Part model, mm, in its own coordinate system. Face numbers are marked on the shaded views. A direction names the side the tool comes from. Give positions to 0.01 mm unless a question says otherwise; leave off trailing zeros. Order: outer loops, then holes, each group sorted by start corner. A loop starts at its lowest first (then second) coordinate and runs counter-clockwise, first axis right, second up.
1. Slice it at C-C on z = 6.75. List the corners of the cut face in (x, y), and give its area (3 significant figures).
2. Slice it at A-A on y = 0. List the corners of the cut face in (x, z).
3. Slice it at B-B on x = 38. List the corners of the cut face in (y, z), and give its area (3 significant figures).
4. Probe line 1 (Y direction, x = 43.5, z = 24.5); line 2 (Z direction, x = 40.5, y = 1.55); line 3 (Z direction, x = 48, y = -2.25). List the from-to ranges inside material, lowest first.
5. Which spindle directions (+Z, -Z, +X, -X, +Y, -Y) get a long thin tool onto all of the face, cutting with end or side? Do the marked faces 1 and 2. Say none if no direction does.
6. Drop flat-ended pins along their axis: pin 1 Ø3 at (y, z) = (1.5, 11) entering from -X; pin 2 Ø3 at (y, z) = (-1.5, 17) entering from +X; pin 3 Ø3 at (x, y) = (14.5, 1.5) entering from +Z. Give the stop position or say it passes through.
from build123d import *

# Parameters (mm, degrees)
F1_R     = 2.5
F3_SIZE2 = 0.5
F3_SIZE  = 0.5


with BuildPart() as f2:
    # F2: sweep along a path in F0
    with BuildLine(Plane.XZ) as f2_path:
        Line((0, 0), (0, 10))
        ThreePointArc((0, 10), (4.686291501, 21.313708499), (16, 26))
        Line((16, 26), (96, 26))
    # F1 (on Top) → F2 (sweep)
    with BuildSketch(Plane.XY):
        Circle(F1_R)
    sweep(path=f2_path.line)

    # F3
    f3_edges = [f2.edges().sort_by_distance(p)[0] for p in [
        (-2.5, 0, 0),
        (96, 0, 28.5),
    ]]
    chamfer(f3_edges, length=F3_SIZE, length2=F3_SIZE2)


solid = f2.part
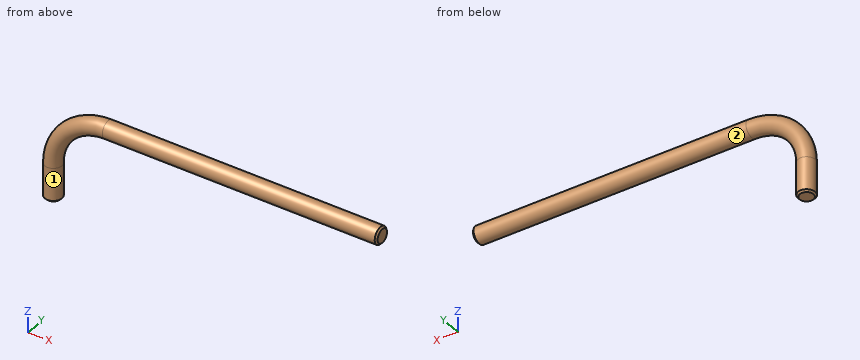
Data:
1. outline: circle Ø5 at (0, 0)
1. area: 19.6 mm2
2. outline: (-2.5, 0.5) - (-2, 0) - (2, 0) - (2.5, 0.5) - (2.5, 10) arc R13.5 cw to (16, 23.5) - (95.5, 23.5) - (96, 24) - (96, 28) - (95.5, 28.5) - (16, 28.5) arc R18.5 ccw to (-2.5, 10) - close
3. outline: circle Ø5 at (0, 26)
3. area: 19.6 mm2
4. line 1: y = -2 to 2
4. line 2: z = 24.04 to 27.96
4. line 3: z = 24.91 to 27.09
5. face 1: -Z
5. face 2: +X
6. pin 1: stops at x = -2.49
6. pin 2: stops at x = 5.21
6. pin 3: stops at z = 28.48
